The model under review builds one solid part; all positions refer to its coordinate system, in mm. A direction names the side the tool comes from. Give positions to 0.01 mm unless a question says otherwise; leave off trailing zeros. Order: outer loops, then holes, each group sorted by start corner. A loop starts at its lowest first (then second) coordinate and runs counter-clockwise, first axis right, second up. Notation, with made-up numbers: (15.5, -29.75) - (19.5, -29.75) arc R5 cw to (19.5, -20.75) - close; hole circle Ø7 at (27, -38). An arc over 180 degrees is marked (long way). Put each result on its own line as item: value.
```python
from build123d import *

# Parameters (mm, degrees)
F0_W     = 90
F0_H     = 60
F1_DEPTH = 58
F2_W     = 90
F2_H     = 60
F3_DEPTH = 55
F4_DEPTH = 55


with BuildPart() as f1:
    # F0 (on Top) → F1 (new body)
    with BuildSketch(Plane.XY):
        Polygon((55, 33), (48, 33), (-48, 33), (-55, 33), (-55, -33), (-48, -33), (48, -33), (55, -33), align=None)
        Rectangle(F0_W, F0_H, mode=Mode.SUBTRACT)
        Rectangle(F0_W, F0_H)
    extrude(amount=F1_DEPTH)

    # F2 (on face) → F3 (join)
    with BuildSketch(Plane.XY.offset(58)):
        Rectangle(F2_W, F2_H)
    extrude(amount=-F3_DEPTH)

    # F2 (on face) → F4 (cut)
    with BuildSketch(Plane.XY.offset(58)):
        Rectangle(F2_W, F2_H)
    extrude(amount=-F4_DEPTH, mode=Mode.SUBTRACT)


solid = f1.part
```
(1) Wall thickness on L1, parallel to Y at x = 36, z = 26; L2, parallel to X at y = -21.5, z = 31; L3, parallel to Z at x = 43, y = -29: over which ranges is each line inside the solid? List them lowest first.
The answers:
L1: -33 to -30, 30 to 33
L2: -55 to -45, 45 to 55
L3: 0 to 3
(2) Take a section at A-A, the plane z = 37.5. Write out the cut boundary in (x, y).
The answers:
outline: (-55, -33) - (55, -33) - (55, 33) - (-55, 33) - close; hole (-45, -30) - (45, -30) - (45, 30) - (-45, 30) - close
(3) Take a section at C-C, the plane x = 3.5. Write out the cut boundary in (y, z).
The answers:
outline: (-33, 0) - (33, 0) - (33, 58) - (30, 58) - (30, 3) - (-30, 3) - (-30, 58) - (-33, 58) - close
(4) Take a section at B-B, the plane y = -0.5. Write out the cut boundary in (x, z).
The answers:
outline: (-55, 0) - (55, 0) - (55, 58) - (45, 58) - (45, 3) - (-45, 3) - (-45, 58) - (-55, 58) - close
(5) The part is to be moulded in two halves that separate along Y. For faces 1 (the flat face through (-1, -33, 29)), 2 (the flat face through (-45, 0, 31)), 3 (the flat face through (-8, 32, 58)), say which applies: pulls with the +Y half, pulls with the -Y half, needs draft (parallel to the pull), parting line crosses it, or undercut.
The answers:
face 1: pulls with the -Y half
face 2: undercut
face 3: needs draft
(6) For faces 4 (the flat face through (-1, -30, 31)), 5 (the flat face through (55, 0, 29)), list the 3-axis set-ups (+Z, -Z, +X, -X, +Y, -Y) from which the entire face can be reached by the end or side of a thin tool; tool diameter is ignored.
The answers:
face 4: +Z
face 5: +Z, -Z, +X, +Y, -Y
(7) Clearance check with a flat-ended pin moving along its axis: pin 1 Ø2 at (x, y) = (43.5, 21) entering from +Z. State where the tip first meets the part, or that it passes through.
The answers:
pin 1: z = 3
